Input: part model. Units: mm. Frame: model coordinates. Give positions to 0.01 mm unless a question says otherwise; leave off trailing zeros. Loops run counter-clockwise (first coordinate to the right, second up) from the corner with the lowest first, then second, coordinate; pieces in that order, holes last. Notation, with made-up numbers: (-10, 45.25) -> (23, 45.25) arc R23 ccw to (23, 81.25) -> close; hole circle Ø5 at (5, -15). An arc over 180 degrees is marked (long way). Answer in a Markdown table with one row per item. Add a question column.
```python
from build123d import *

# Parameters (mm, degrees)
SKETCH1_R               = 88.9
SKETCH1_R_2             = 85.725
BOSS_EXTRUDE1_DEPTH     = 203.581
CUT_EXTRUDE1_REACH      = 241.273
CUT_EXTRUDE1_END_RADIUS = 88.9
SKETCH2_W               = 127
SKETCH2_H               = 356.362
CIRPATTERN1_COUNT       = 3


with BuildPart() as part:
    # Sketch1 → Boss-Extrude1 (new, symmetric)
    with BuildSketch(Plane(origin=(0, 0, 0), x_dir=(1, 0, 0), z_dir=(0, 1, 0))):
        with Locations(Location((0, 0, 0), (0, 0, 270))):
            Circle(SKETCH1_R)
        with Locations(Location((0, 0, 0), (0, 0, 270))):
            Circle(SKETCH1_R_2, mode=Mode.SUBTRACT)
    extrude(amount=BOSS_EXTRUDE1_DEPTH, both=True)

    # Cut-Extrude1: up to this cylinder (the profile starts inside it)
    cut_extrude1_end = Plane(origin=(0, 0, 0), z_dir=(0, -1, 0)) * Cylinder(CUT_EXTRUDE1_END_RADIUS, 661.346, mode=Mode.PRIVATE)
    # Sketch2 → Cut-Extrude1 (cut, up to the surface)
    with BuildSketch(Plane.XY, mode=Mode.PRIVATE) as cut_extrude1_sk1:
        Rectangle(SKETCH2_W, SKETCH2_H)
    cut_extrude1_tool1 = extrude(cut_extrude1_sk1.sketch, amount=-CUT_EXTRUDE1_REACH, mode=Mode.PRIVATE) & cut_extrude1_end
    cut_extrude1 = cut_extrude1_tool1.solids().sort_by_distance((0, 0, 0))[0]
    add(cut_extrude1, mode=Mode.SUBTRACT)

    # CirPattern1: Cut-Extrude1 ×3 about axis
    cirpattern1_axis = Axis((0, 0, 0), (0, 1, 0))
    for i in range(1, CIRPATTERN1_COUNT):
        add(cut_extrude1.rotate(cirpattern1_axis, i * 360 / CIRPATTERN1_COUNT), mode=Mode.SUBTRACT)


solid = part.part
```
1) Section B-B on y = -46. Output: boundary loops of the cut face in (x, z) (3 decimals), and give its area (3 significant figures).
2) Pull-direction query (X, two-part tool) for faces 1 (the face through (73, -203.581, -47)), 2 (the face through (9.03, 0.95, 88.44)), 3 (the face through (8.703, -0.95, 85.282)); classes: +X half, -X half, draft (parallel to the pull), parting line (faces both ways), or undercut.
3) Pin query (flat end, axial travel): pin 1 (10 mm diameter, centred on x = 29.5, y = 156, fed in from +Z); pin 2 (1.5 mm diameter, centred on y = -50, z = -58.5, fed in from -X); pin 3 (8 mm diameter, centred on y = 34, z = -52, fed in from -X); pin 4 (1.4 mm diameter, centred on y = -6, z = -61, fed in from -X). Return the tip coordinate at first contact, or that it passes through.
4) Section D-D on x = 26.5. Output: boundary loops of the cut face in (y, z).
5) Material intervals for line 1 along Z through (x, y) = (0, 39.5) (3 decimals); line 2 along Z through (x, y) = (-3, -171.5), sorted ascending.
6) Section A-A on x = 0. Output: boundary loops of the cut face in (y, z) (3 decimals).
7) Section C-C on z = 0. Output: boundary loops of the cut face in (x, y) (3 decimals).
Working result:
| question | item | result |
|---|---|---|
| 1 | outline | (-85.632, -23.884) arc R88.9 ccw to (-63.5, -62.217) -> (-63.5, -57.589) arc R85.725 cw to (-81.624, -26.198) -> close; (-22.132, 86.101) -> (-18.124, 83.787) arc R85.725 cw to (18.124, 83.787) -> (22.132, 86.101) arc R88.9 ccw to start; (63.5, -62.217) arc R88.9 ccw to (85.632, -23.884) -> (81.624, -26.198) arc R85.725 cw to (63.5, -57.589) -> close |
| 1 | area | 387 mm2 |
| 2 | face 1 | draft |
| 2 | face 2 | parting line |
| 2 | face 3 | undercut |
| 3 | pin 1 | passes through |
| 3 | pin 2 | stops at x = -67.59 |
| 3 | pin 3 | stops at x = -74.83 |
| 3 | pin 4 | stops at x = -65.32 |
| 4 | outline | (-203.58, -84.86) -> (-178.18, -84.86) -> (-178.18, -81.53) -> (-203.58, -81.53) -> close; (-203.58, 81.53) -> (-178.18, 81.53) -> (-178.18, 84.86) -> (-203.58, 84.86) -> close; (178.18, -84.86) -> (203.58, -84.86) -> (203.58, -81.53) -> (178.18, -81.53) -> close; (178.18, 81.53) -> (203.58, 81.53) -> (203.58, 84.86) -> (178.18, 84.86) -> close |
| 5 | line 1 | z = 85.725 to 88.9 |
| 5 | line 2 | z = 85.67 to 88.85 |
| 6 | outline | (-203.581, -88.9) -> (-178.181, -88.9) -> (-178.181, -85.725) -> (-203.581, -85.725) -> close; (-203.581, 85.725) -> (203.581, 85.725) -> (203.581, 88.9) -> (-203.581, 88.9) -> close; (178.181, -88.9) -> (203.581, -88.9) -> (203.581, -85.725) -> (178.181, -85.725) -> close |
| 7 | outline | (-88.9, -203.581) -> (-85.725, -203.581) -> (-85.725, -178.181) -> (-88.9, -178.181) -> close; (-88.9, 178.181) -> (-85.725, 178.181) -> (-85.725, 203.581) -> (-88.9, 203.581) -> close; (85.725, -203.581) -> (88.9, -203.581) -> (88.9, -178.181) -> (85.725, -178.181) -> close; (85.725, 178.181) -> (88.9, 178.181) -> (88.9, 203.581) -> (85.725, 203.581) -> close |
